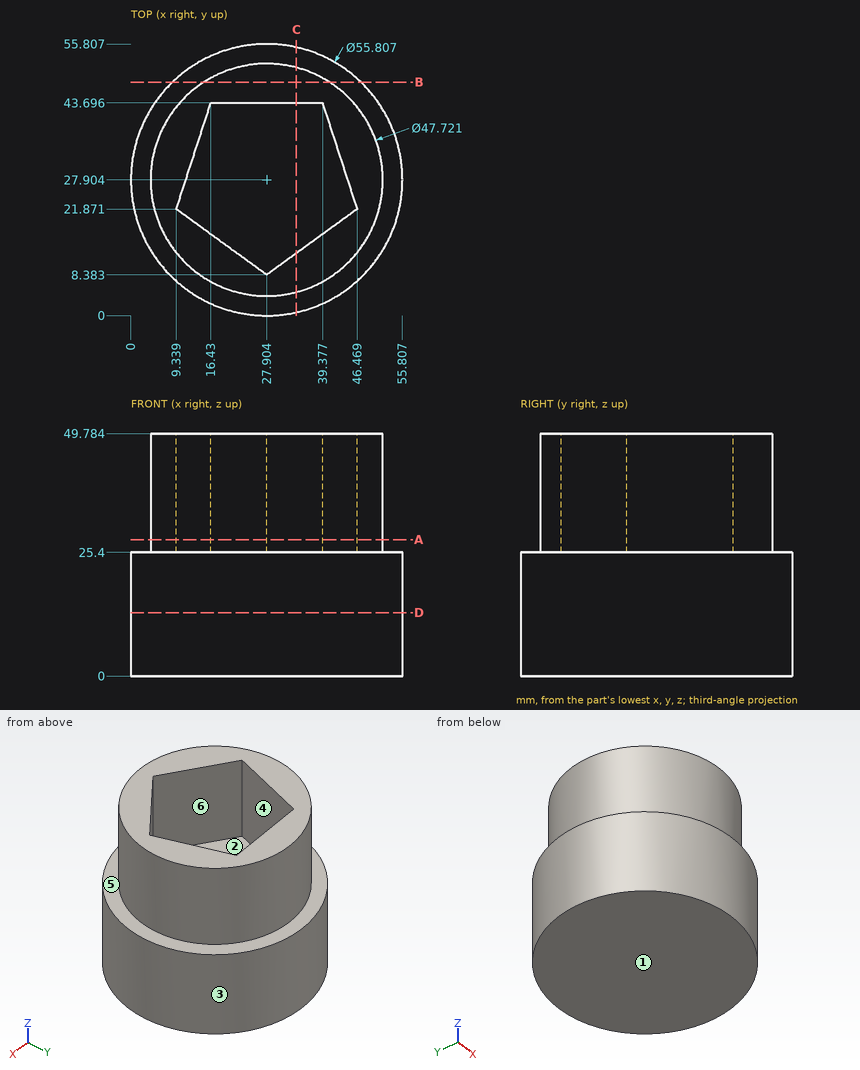
For this review, use the dimensioned drawing (mm, ordinates from the lowest corner) and the shaded views. A direction names the side the tool comes from. Round coordinates to 2 decimals unless told otherwise and drop trailing zeros. Order: outer loops, then holes, each group sorted by start corner. A loop starts at its lowest first (then second) coordinate and runs counter-clockwise, first axis right, second up.
1) Machinability: for the marked faces 1 and 2, which of the approach directions +Z, -Z, +X, -X, +Y, -Y give a long, thin tool a straight path to every point of the face, cutting with its end or side? Answer none if there is none.
The answers:
face 1: -Z, +X, -X, +Y, -Y
face 2: +Z
2) Clearance check with flat-ended pins moving along their axes: pin 1 Ø3 at (x, y) = (11, 45) entering from +Z; pin 2 Ø10 at (x, z) = (30, 29.5) entering from -Y; pin 3 Ø2 at (y, z) = (31, 39) entering from -X (1 decimal); pin 4 Ø1 at (x, y) = (13.5, 20.5) entering from +Z. State where each tip first meets the part, or that it passes through.
The answers:
pin 1: stops at z = 49.78
pin 2: stops at y = 0
pin 3: stops at x = 4.1
pin 4: stops at z = 25.4
3) Consider section D-D (z = 13). State the section outline as (x, y) points.
The answers:
outline: circle Ø55.81 at (27.9, 27.9)
4) Draft analysis for pull direction X (two halves, no side actions). For the marked faces 3, 4, 5 and 6, state which applies: released by +X, released by -X, zero draft, split by the parting line, or undercut.
The answers:
face 3: split by the parting line
face 4: undercut
face 5: zero draft
face 6: undercut
5) Consider section B-B (y = 48). State the section outline as (x, z) points (1 decimal), plus the area to 3 significant figures.
The answers:
outline: (8.5, 0) - (47.3, 0) - (47.3, 25.4) - (40.8, 25.4) - (40.8, 49.8) - (15, 49.8) - (15, 25.4) - (8.5, 25.4) - close
area: 1,610 mm2
6) Consider section C-C (x = 34). State the section outline as (y, z) points (1 decimal), plus the area to 4 significant figures.
The answers:
outline: (0.7, 0) - (55.1, 0) - (55.1, 25.4) - (51, 25.4) - (51, 49.8) - (43.7, 49.8) - (43.7, 25.4) - (12.8, 25.4) - (12.8, 49.8) - (4.8, 49.8) - (4.8, 25.4) - (0.7, 25.4) - close
area: 1,755 mm2
7) For L1, parallel to Z at x = 44, y = 21.5; L2, parallel to X at y = 14, z = 39 (1 decimal); L3, parallel to Y at x = 27, z = 42 (1 decimal), list the stretches that pass through material, from the lowest coordinate up.
The answers:
L1: z = 0 to 25.4
L2: x = 8.5 to 20.2, 35.6 to 47.3
L3: y = 4.1 to 9, 43.7 to 51.7
8) Consider section A-A (z = 28). State the section outline as (x, y) points (1 decimal).
The answers:
outline: circle Ø47.7 at (27.9, 27.9); hole (9.3, 21.9) - (27.9, 8.4) - (46.5, 21.9) - (39.4, 43.7) - (16.4, 43.7) - close
